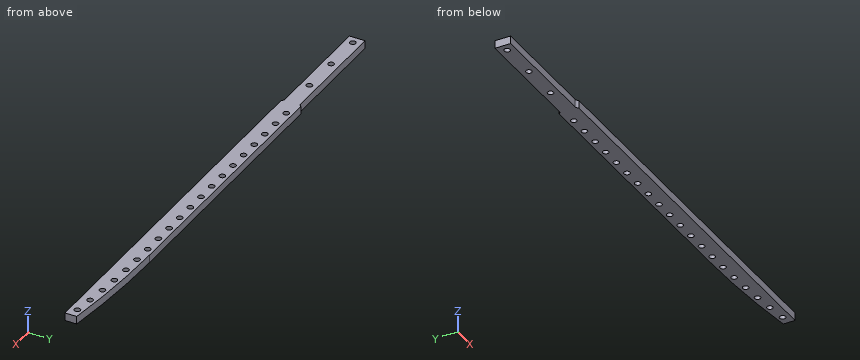
from build123d import *

# Parameters (mm, degrees)
SKETCH_1_W                = 260
SKETCH_1_H                = 10
EXTRUDE_1_DEPTH           = 4
SKETCH_2_W                = 122
SKETCH_2_H                = 2
CUT_EXTRUDE_1_DEPTH       = 4
SKETCH_4_R                = 1.5
CUT_EXTRUDE_2_DEPTH       = 4
FILLET_1_R                = 2
SKETCH_7_R                = 1.5
CUT_EXTRUDE_3_DEPTH       = 4
PATTERN_CURVE_1_OUTLINE_R = 1.5
PATTERN_CURVE_1_DEPTH     = 4
CUT_EXTRUDE_4_DEPTH       = 4


# Read off the part's stored shape, not the designer's step: 曲线阵列1
with BuildPart() as part:
    # 草图1 → 凸台-拉伸1 (new body)
    with BuildSketch(Plane.XY):
        Rectangle(SKETCH_1_W, SKETCH_1_H)
    extrude(amount=EXTRUDE_1_DEPTH)

    # 草图2 → 切除-拉伸1 (cut)
    with BuildSketch(Plane.XY.offset(4)):
        with Locations((-130, 5)):
            Rectangle(SKETCH_2_W, SKETCH_2_H)
    cut_extrude_1 = extrude(amount=-CUT_EXTRUDE_1_DEPTH, mode=Mode.SUBTRACT)

    # 镜向1: 切除-拉伸1 across plane
    add(cut_extrude_1.mirror(Plane.ZX), mode=Mode.SUBTRACT)

    # 草图4 → 切除-拉伸2 (cut)
    with BuildSketch(Plane.XY.offset(4)):
        with Locations((-126, 0)):
            Circle(SKETCH_4_R)
        with Locations((-86, 0)):
            Circle(SKETCH_4_R)
        with Locations((-106, 0)):
            Circle(SKETCH_4_R)
    extrude(amount=-CUT_EXTRUDE_2_DEPTH, mode=Mode.SUBTRACT)

    # 圆角1
    # the kernel refuses this fillet: 2 mm, written as the material it adds along each edge
    with BuildSketch(Plane(origin=(-69, -4, 4), x_dir=(0, -1, 0), z_dir=(0, 0, -1))) as fillet_1_piece_1:
        with BuildLine():
            CenterArc((2, 1.732050808), FILLET_1_R, 180, 60)
            Line((0, 1.732050808), (-0.04, 1.732050808))
            Line((-0.04, 1.732050808), (-0.04, 0))
            Line((-0.04, 0), (0, -0.04))
            ThreePointArc((0, -0.04), (0.5, -0.04), (0.98, -0.034641016))
            Line((0.98, -0.034641016), (1, 0))
        make_face()
    extrude(amount=4)
    with BuildSketch(Plane(origin=(-69, 4, 4), x_dir=(-1, 0, 0), z_dir=(0, 0, -1))) as fillet_1_piece_2:
        with BuildLine():
            CenterArc((1.732050808, 2), FILLET_1_R, 210, 60)
            Line((0, 1), (-0.034641016, 0.98))
            ThreePointArc((-0.034641016, 0.98), (-0.04, 0.5), (-0.04, 0))
            Line((-0.04, 0), (0, -0.04))
            Line((0, -0.04), (1.732050808, -0.04))
            Line((1.732050808, -0.04), (1.732050808, 0))
        make_face()
    extrude(amount=4)

    # 草图7 → 切除-拉伸3 (cut)
    with BuildSketch(Plane.XY.offset(4)):
        with Locations((-61, 2)):
            Circle(SKETCH_7_R)
    extrude(amount=-CUT_EXTRUDE_3_DEPTH, mode=Mode.SUBTRACT)

    # 曲线阵列1 outline → 曲线阵列1 (cut)
    with BuildSketch(Plane.XY):
        with Locations((125.062891226, -1.366432364)):
            Circle(PATTERN_CURVE_1_OUTLINE_R)
        with Locations((115.323700734, -0.278128004)):
            Circle(PATTERN_CURVE_1_OUTLINE_R)
        with Locations((105.563205139, 0.598777673)):
            Circle(PATTERN_CURVE_1_OUTLINE_R)
        with Locations((95.785992512, 1.263872463)):
            Circle(PATTERN_CURVE_1_OUTLINE_R)
        with Locations((85.996658783, 1.716843728)):
            Circle(PATTERN_CURVE_1_OUTLINE_R)
        with Locations((76.199805579, 1.957478543)):
            Circle(PATTERN_CURVE_1_OUTLINE_R)
        with Locations((66.4, 2)):
            Circle(PATTERN_CURVE_1_OUTLINE_R)
        with Locations((56.6, 2)):
            Circle(PATTERN_CURVE_1_OUTLINE_R)
        with Locations((46.8, 2)):
            Circle(PATTERN_CURVE_1_OUTLINE_R)
        with Locations((37, 2)):
            Circle(PATTERN_CURVE_1_OUTLINE_R)
        with Locations((27.2, 2)):
            Circle(PATTERN_CURVE_1_OUTLINE_R)
        with Locations((17.4, 2)):
            Circle(PATTERN_CURVE_1_OUTLINE_R)
        with Locations((7.6, 2)):
            Circle(PATTERN_CURVE_1_OUTLINE_R)
        with Locations((-2.2, 2)):
            Circle(PATTERN_CURVE_1_OUTLINE_R)
        with Locations((-12, 2)):
            Circle(PATTERN_CURVE_1_OUTLINE_R)
        with Locations((-21.8, 2)):
            Circle(PATTERN_CURVE_1_OUTLINE_R)
        with Locations((-31.6, 2)):
            Circle(PATTERN_CURVE_1_OUTLINE_R)
        with Locations((-41.4, 2)):
            Circle(PATTERN_CURVE_1_OUTLINE_R)
        with Locations((-51.2, 2)):
            Circle(PATTERN_CURVE_1_OUTLINE_R)
    extrude(amount=PATTERN_CURVE_1_DEPTH, mode=Mode.SUBTRACT)

    # 草图8 → 切除-拉伸4 (cut)
    with BuildSketch(Plane.XY.offset(4)):
        with BuildLine():
            Line((70, 5), (130, 5))
            Line((130, 5), (130.398230088, 0.973451327))
            ThreePointArc((130.398230088, 0.973451327), (100.266149788, 3.992246825), (70, 5))
        make_face()
    extrude(amount=-CUT_EXTRUDE_4_DEPTH, mode=Mode.SUBTRACT)


solid = part.part
Source: CAD feature listing. Evaluate the final solid. Frame: model axes, mm. Coordinates: 2 decimals unless noted, no trailing zeros. Loops run counter-clockwise (first coordinate to the right, second up) from the corner with the lowest first, then second, coordinate; pieces in that order, holes last. Notation, with made-up numbers: (79, 22) - (104, 22) arc R5 ccw to (104, 31) - close; hole circle Ø9 at (13.5, 45). An arc over 180 degrees is marked (long way). One line per item, written item: value. Start each with the question number.
1. Section A-A (z = 2.4). State how many separate pieces and enclosed holes the cut face has, and give its area (3 significant figures).
2. Ray query, L1, parallel to Y at x = 17.4, z = 2.6; L2, parallel to Y at x = -86, z = 1.15; L3, parallel to Y at x = -90.5, z = 2.05. Return the intervals inside material, ascending.
3. Contact query for a flat-ended pin moving along its axis: P1, Ø2, axis at x = -93.5, z = 3, coming from the -Y side. Output: stop coordinate, or through.
4. Section B-B (x = -100). Return the cut outline in (y, z), and give its area (3 significant figures).
Verdict:
1. separate pieces: 1
1. enclosed holes: 23
1. area: 2,240 mm2
2. L1: y = -5 to 0.5, 3.5 to 5
2. L2: y = -4 to -1.5, 1.5 to 4
2. L3: y = -4 to 4
3. P1: stops at y = -4
4. outline: (-4, 0) - (4, 0) - (4, 4) - (-4, 4) - close
4. area: 32.0 mm2
